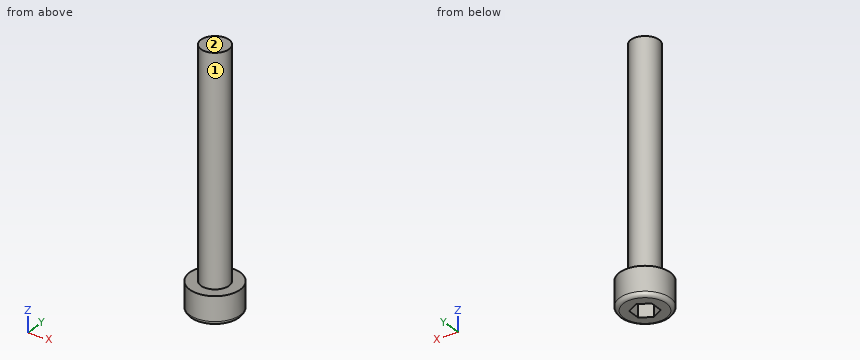
```python
from build123d import *

# Parameters (mm, degrees)
CROQUIS1_R              = 1.25
SALIENTE_EXTRUIR1_DEPTH = 20
CROQUIS2_R              = 2.25
SALIENTE_EXTRUIR2_DEPTH = 2.5
CORTAR_EXTRUIR1_DEPTH   = 1.5
REDONDEO1_R             = 0.35


with BuildPart() as part:
    # Croquis1 → Saliente-Extruir1 (new body)
    with BuildSketch(Plane.XY):
        Circle(CROQUIS1_R)
    extrude(amount=SALIENTE_EXTRUIR1_DEPTH)

    # Croquis2 → Saliente-Extruir2 (add)
    with BuildSketch(Plane(origin=(0, 0, 0), x_dir=(-1, 0, 0), z_dir=(0, 0, -1))):
        Circle(CROQUIS2_R)
    extrude(amount=SALIENTE_EXTRUIR2_DEPTH)

    # Croquis3 → Cortar-Extruir1 (cut)
    with BuildSketch(Plane(origin=(0, 0, -2.5), x_dir=(-1, 0, 0), z_dir=(0, 0, -1))):
        Polygon((0, -1.154700538), (1, -0.577350269), (1, 0.577350269), (0, 1.154700538), (-1, 0.577350269), (-1, -0.577350269), align=None)
    extrude(amount=-CORTAR_EXTRUIR1_DEPTH, mode=Mode.SUBTRACT)

    # Redondeo1
    redondeo1_edges = [part.edges().sort_by_distance(p)[0] for p in [
        (2.25, 0, -2.5),
    ]]
    fillet(redondeo1_edges, radius=REDONDEO1_R)


solid = part.part
```
The listing builds one solid part. Answer for the finished solid, in the listing's coordinates (mm). Face numbers are marked on the shaded views. A direction names the side the tool comes from. Round coordinates to 2 decimals unless told otherwise and drop trailing zeros. Order: outer loops, then holes, each group sorted by start corner. A loop starts at its lowest first (then second) coordinate and runs counter-clockwise, first axis right, second up. Notation, with made-up numbers: (78, 1.25) -> (104, 1.25) arc R7 ccw to (104, 9.25) -> close; hole circle Ø7 at (76.5, 89). An arc over 180 degrees is marked (long way). Answer as CSV lines item,"result". Start each with the question number.
(1) Find the intervals of material crossed by probe 1 along Y at (x, z) = (0.75, 6.25); probe 2 along Z at (x, y) = (0.55, -1.25); probe 3 along Y at (x, z) = (0, 1), in increasing order. Write a range as from..to.
(2) The part is cut by section A-A (y = 0). Determine the outline of the cut face in (x, z), then the cut area to 3 significant figures.
(3) A tool of negligible diameter and unlimited length cuts with its end or side. For the marked faces 1 and 2, from which of +Z, -Z, +X, -X, +Y, -Y can it reach the whole face along a straight path? Write none if from no direction.
(4) Flat-ended cylindrical pins translate along their axes: pin 1 Ø2 at (y, z) = (0.5, 9) entering from -X; pin 2 Ø1 at (y, z) = (-1.5, 17) entering from +X. Find the tip coordinate at first contact, or state that the pin passes through.
(5) The part is cut by section B-B (z = 4.25). Determine the outline of the cut face in (x, y).
Evaluation:
1,probe 1,"-1..1"
1,probe 2,"-2.5..0"
1,probe 3,"-1.25..1.25"
2,outline,"(-2.25, -2.15) arc R0.35 ccw to (-1.9, -2.5) -> (-1, -2.5) -> (-1, -1) -> (1, -1) -> (1, -2.5) -> (1.9, -2.5) arc R0.35 ccw to (2.25, -2.15) -> (2.25, 0) -> (1.25, 0) -> (1.25, 20) -> (-1.25, 20) -> (-1.25, 0) -> (-2.25, 0) -> close"
2,area,"58.2 mm²"
3,face 1,"+Z"
3,face 2,"+Z, +X, -X, +Y, -Y"
4,pin 1,"x = -1.25"
4,pin 2,"x = 0.75"
5,outline,"circle Ø2.5 at (0, 0)"
